Part model, mm, in its own coordinate system. A direction names the side the tool comes from. Give positions to 0.01 mm unless a question says otherwise; leave off trailing zeros. Order: outer loops, then holes, each group sorted by start corner. A loop starts at its lowest first (then second) coordinate and runs counter-clockwise, first axis right, second up. Notation, with made-up numbers: M -36,41.5 L -26,41.5 A34 cw -26,71.5 Z; hole C 42,-36.75 d8. An arc over 180 degrees is marked long. Return JSON: item names as keys, results as strings.
Autodesk Fusion 360 part; units mm, degrees
sketch "スケッチ1" plane through (0, 0, 0) normal (0, 0, 1) x (1, 0, 0)
  line L0 (-9.5, 140) -> (-80.5, 140)
  line L1 (-80.5, 140) -> (-80.5, -140)
  line L2 (-80.5, -140) -> (-9.5, -140)
  line L3 (80.5, -25) -> (80.5, 130)
  line L4 (74.75, 130) -> (-80.5, -140) construction
  line L5 (-80.5, 140) -> (42.3815, -73.707) construction
  line L6 (-9.5, 140) -> (-9.5, 130)
  line L7 (-9.5, 130) -> (80.5, 130)
  line L8 (-80.5, -140) -> (-9.5, -140) construction
  line L9 (80.5, -25) -> (-9.5, -140)
  dimension "d2" = 280
  dimension "d5" = 71
extrude "押し出し1" add sketch "スケッチ1" along normal blind 6
chamfer "面取り1" distance 25 angle 45 2 edges at (-80.5, -140, 3) (-80.5, 140, 3)
sketch "スケッチ2" plane through (0, 0, 6) normal (0, 0, 1) x (-1, 0, 0)
  line L0 (55.5, -140) -> (80.5, -115)
  line L1 (80.5, -115) -> (80.5, 115)
  line L2 (80.5, 115) -> (55.5, 140)
  line L3 (55.5, 140) -> (9.5, 140)
  line L4 (9.5, 140) -> (-80.5, 25)
  line L5 (-80.5, 25) -> (-80.5, -130)
  line L6 (-80.5, -130) -> (9.5, -130)
  line L7 (9.5, -130) -> (9.5, -140)
  line L8 (9.5, -140) -> (55.5, -140)
  line L9 (-80.5, -130) -> (-40.5, -130) construction
  line L10 (-40.5, -130) -> (-40.5, -90) construction
  line L11 (-40.5, -90) -> (-80.5, -90) construction
  line L12 (-80.5, -90) -> (-80.5, -130) construction
  line L13 (-40.5, -90) -> (-40.5, -35) construction
  point P0 (-40.5, -90)
  point P1 (-40.5, -35)
  dimension "d10" = 40
  dimension "d11" = 40
  dimension "d12" = 55
hole "穴1" at (40.5, 90, 6) at (40.5, 35, 6) direction (0, 0, -1) diameter 18 end through all
equation "d5 = 25 mm + 46 mm"
Q1. Pin check, flat tip, straight feed: pin 1 (1.8 mm diameter, centred on y = 134.5, z = 2.5, fed in from +X). Stop position of the tip, or through.
Established:
{"pin 1": "stops at x = -9.5"}
Q2. Band-saw the part on B-B (z = 2.55). Give the cut face in (x, y), then the cut area to 3 significant figures.
Established:
{"outline": "M -80.5,-115 L -55.5,-140 L -9.5,-140 L 80.5,-25 L 80.5,130 L -9.5,130 L -9.5,140 L -55.5,140 L -80.5,115 Z; hole C 40.5,35 d18; hole C 40.5,90 d18", "area": "37,900 mm²"}
Q3. Band-saw the part on D-D (y = -56.5). Give the cut face in (x, z), then the cut area to 3 significant figures.
Established:
{"outline": "M -80.5,0 L 55.85,0 L 55.85,6 L -80.5,6 Z", "area": "818 mm²"}
Q4. 3-axis set-ups, long thin cutter, end or side, ignore diameter. For faces 4 (the flat face through (-1, 2, 6)), 5 (the flat face through (35, 130, 3)): which of +Z, -Z, +X, -X, +Y, -Y reach the whole face in a straight line?
Established:
{"face 4": "+Z, +X, -X, +Y, -Y", "face 5": "+Z, -Z, +X, +Y"}
Q5. Two-plate mould, pull along Y, no slides. Class faces 1 (the flat face through (-32, 140, 3)), 2 (the flat face through (-1, 2, 0)), 3 (the cylindrical face through (34.417, 41.633, 2.958)): +Y half, -Y half, draft (parallel to the pull), parting line (faces both ways), or undercut.
Established:
{"face 1": "+Y half", "face 2": "draft", "face 3": "undercut"}
Q6. Band-saw the part on A-A (y = 35). Give the cut face in (x, z), then the cut area to 3 significant figures.
Established:
{"outline": "M -80.5,0 L 31.5,0 L 31.5,6 L -80.5,6 Z; M 49.5,0 L 80.5,0 L 80.5,6 L 49.5,6 Z", "area": "858 mm²"}
Q7. Probe line 1 along Y through (x, z) = (40.5, 2.7); line 2 along Y through (x, z) = (37, 2.3); line 3 along X through (y, z) = (90, 1.85). List the from-to ranges inside material, lowest first.
Established:
{"line 1": "y = -76.11 to 26, 44 to 81, 99 to 130", "line 2": "y = -80.58 to 26.71, 43.29 to 81.71, 98.29 to 130", "line 3": "x = -80.5 to 31.5, 49.5 to 80.5"}
Q8. Band-saw the part on C-C (x = 40.5). Give the cut face in (y, z), then the cut area to 3 significant figures.
Established:
{"outline": "M -76.11,0 L 26,0 L 26,6 L -76.11,6 Z; M 44,0 L 81,0 L 81,6 L 44,6 Z; M 99,0 L 130,0 L 130,6 L 99,6 Z", "area": "1,020 mm²"}
